Here's how the part is built. I have some questions about the finished solid (model axes, mm). A direction names the side the tool comes from. Coordinates: 2 decimals unless noted, no trailing zeros. Write each loop counter-clockwise with the first axis right and the second up, starting at its lowest first coordinate (ties: lowest second). Pieces come first, ordered by that corner, then holes.
from build123d import *

# Parameters (mm, degrees)
REVOLUTION_ANGLE = -180
SKETCH001_R      = 1.6
POCKET_DEPTH     = 5
SKETCH002_R      = 3.25
PAD_DEPTH        = 3
SKETCH003_W      = 2
SKETCH003_H      = 10
PAD001_DEPTH     = 9.8
SKETCH004_R      = 1.6
POCKET001_DEPTH  = 5


with BuildPart() as part:
    # Sketch → Revolution (revolve, symmetric)
    with BuildSketch(Plane.XZ) as revolution_sk:
        Polygon((4.5, 20), (8.5, 20), (14.5, 16), (14.5, 0), (16.5, 0), (16.5, 5), (26.5, 5), (26.5, 7), (16.5, 7), (16.5, 16.821367), (10.232051, 21), (4.5, 21), align=None)
    revolve(axis=Axis((0, 0, 0), (0, 0, 1)), revolution_arc=REVOLUTION_ANGLE / 2)
    revolve(revolution_sk.sketch, axis=Axis((0, 0, 0), (0, 0, -1)), revolution_arc=REVOLUTION_ANGLE / 2)

    # Sketch001 (on Face8 of Revolution) → Pocket (cut)
    with BuildSketch(Plane(origin=(0, 0, 7), x_dir=(-1, 0, 0), z_dir=(0, 0, 1))):
        with Locations((-21, 0)):
            Circle(SKETCH001_R)
        with Locations((-10.5, 18.186533)):
            Circle(SKETCH001_R)
        with Locations((-10.5, -18.186533)):
            Circle(SKETCH001_R)
    extrude(amount=-POCKET_DEPTH, mode=Mode.SUBTRACT)

    # Sketch002 (on Face1 of Pocket) → Pad (join)
    with BuildSketch(Plane(origin=(0, 0, 20), x_dir=(1, 0, 0), z_dir=(0, 0, -1))):
        with Locations((5.628499, 5.4)):
            Circle(SKETCH002_R)
        with Locations((5.628499, -5.4)):
            Circle(SKETCH002_R)
    extrude(amount=PAD_DEPTH)

    # Sketch003 (on Face13 of Pad) → Pad001 (join)
    with BuildSketch(Plane(origin=(0, 0, 7), x_dir=(-1, 0, 0), z_dir=(0, 0, 1))):
        with Locations((-1, 21)):
            Rectangle(SKETCH003_W, SKETCH003_H)
        with Locations((-1, -21)):
            Rectangle(SKETCH003_W, SKETCH003_H)
    extrude(amount=PAD001_DEPTH)

    # Sketch004 (on Face21 of Pad001) → Pocket001 (cut)
    with BuildSketch(Plane(origin=(0, 0, 0), x_dir=(0, 0, -1), z_dir=(-1, 0, 0))):
        with Locations((-12, -21)):
            Circle(SKETCH004_R)
        with Locations((-12, 21)):
            Circle(SKETCH004_R)
    extrude(amount=-POCKET001_DEPTH, mode=Mode.SUBTRACT)


solid = part.part
1. I want a section at A-A (z = 12). List the corners of the cut face in (x, y) for me.
2. I want a section at C-C (y = 21). List the corners of the cut face in (x, z) for me.
3. I want a section at D-D (z = 6.25). List the corners of the cut face in (x, y) for me, then the cut area to 3 significant figures.
4. Thinking about a two-plate mould opening in X: for faces 5 (the face through (19, 0, 7)), 6 (the face through (3.05, -3.42, 18.19)), 7 (the face through (2, 22.3, 10.7)), which applies, pulls with the +X half, pulls with the -X half, needs draft (parallel to the pull), parting line crosses it, or undercut?
5. On a 3-axis mill with a long thin cutter (end or side, diameter ignored), from which of +Z, -Z, +X, -X, +Y, -Y can I reach the whole of each face in a straight line? I mean faces 1 (the face through (16.496, -0.363, 2.535)), 2 (the face through (1, -26, 12)), 3 (the face through (14.496, -0.319, 7.888)), 4 (the face through (16.496, -0.363, 11.979)). Say none if no direction works.
6. For pin 1 Ø7 at (x, y) = (2.5, -1) entering from -Z; pin 2 Ø1 at (x, y) = (12, -9) entering from +Z; pin 3 Ø3.5 at (x, y) = (10.5, 18.19) entering from +Z; pin 4 Ø1.5 at (y, z) = (-15.5, 18.5) entering from +X, each with a flat end and sliding along its axis, tell me the tip position at first contact or that it passes through.
7. I want a section at B-B (x = 20.75). List the corners of the cut face in (y, z) for me, then the cut area to 3 significant figures.
8. If I drill on line 1 (Y direction, x = 10.5, z = 5.55); line 2 (Y direction, x = 1, z = 12); line 3 (Z direction, x = 0.75, y = 21), over which ranges is the centre line in solid material (lowest first)?
Response values:
1. outline: (0, -26) - (2, -26) - (2, -22.6) - (0, -22.6) - close; (0, -19.4) - (2, -19.4) - (2, -16.38) arc R16.5 ccw to (2, 16.38) - (2, 19.4) - (0, 19.4) - (0, 14.5) arc R14.5 cw to (0, -14.5) - close; (0, 22.6) - (2, 22.6) - (2, 26) - (0, 26) - close
2. outline: (0, 5) - (16.16, 5) - (16.16, 7) - (2, 7) - (2, 10.4) - (0, 10.4) - close; (0, 13.6) - (2, 13.6) - (2, 16.8) - (0, 16.8) - close
3. outline: (0, -26.5) arc R26.5 ccw to (0, 26.5) - (0, 14.5) arc R14.5 cw to (0, -14.5) - close; hole circle Ø3.2 at (10.5, -18.19); hole circle Ø3.2 at (10.5, 18.19); hole circle Ø3.2 at (21, 0)
3. area: 749 mm2
4. face 5: needs draft
4. face 6: undercut
4. face 7: pulls with the +X half
5. face 1: -Z, +X
5. face 2: +Z, +X, -X, -Y
5. face 3: -Z, -X
5. face 4: +Z, +X
6. pin 1: stops at z = 17
6. pin 2: stops at z = 18.15
6. pin 3: stops at z = 7
6. pin 4: passes through
7. outline: (-16.48, 5) - (-1.58, 5) - (-1.58, 7) - (-16.48, 7) - close; (1.58, 5) - (16.48, 5) - (16.48, 7) - (1.58, 7) - close
7. area: 59.6 mm2
8. line 1: y = -24.33 to -19.79, -16.59 to -10, 10 to 16.59, 19.79 to 24.33
8. line 2: y = -26 to -22.6, -19.4 to -14.47, 14.47 to 19.4, 22.6 to 26
8. line 3: z = 5 to 10.4, 13.6 to 16.8
